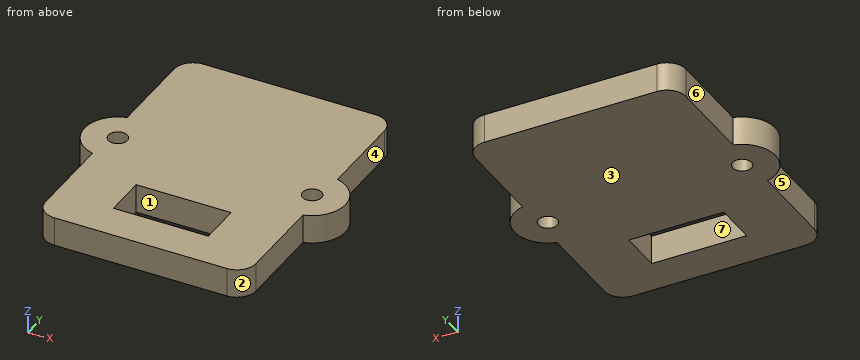
```python
from build123d import *

# Parameters (mm, degrees)
SKETCH2_R           = 1
SKETCH2_W           = 10
SKETCH2_H           = 4.5
BOSS_EXTRUDE2_DEPTH = 3.05


with BuildPart() as part:
    # Sketch2 → Boss-Extrude2 (new body)
    with BuildSketch(Plane.XY):
        with BuildLine():
            Line((-11.075, 15.855524923), (-11.075, 25.133587826))
            ThreePointArc((-11.075, 25.133587826), (-10.489213562, 26.547801388), (-9.075, 27.133587826))
            Line((-9.075, 27.133587826), (9.075, 27.133587826))
            ThreePointArc((9.075, 27.133587826), (10.489213562, 26.547801388), (11.075, 25.133587826))
            Line((11.075, 25.133587826), (11.075, 15.855524923))
            ThreePointArc((11.075, 15.855524923), (13.735, 12.45), (11.075, 9.044475077))
            Line((11.075, 9.044475077), (11.075, -0.233587826))
            ThreePointArc((11.075, -0.233587826), (10.489213562, -1.647801388), (9.075, -2.233587826))
            Line((9.075, -2.233587826), (-9.075, -2.233587826))
            ThreePointArc((-9.075, -2.233587826), (-10.489213562, -1.647801388), (-11.075, -0.233587826))
            Line((-11.075, -0.233587826), (-11.075, 9.044475077))
            ThreePointArc((-11.075, 9.044475077), (-13.735, 12.45), (-11.075, 15.855524923))
        make_face()
        with Locations((-10.225, 12.45)):
            Circle(SKETCH2_R, mode=Mode.SUBTRACT)
        with Locations(Location((10.225, 12.45, 0), (0, 0, 180))):
            Circle(SKETCH2_R, mode=Mode.SUBTRACT)
        with Locations((0, 4.016412174)):
            Rectangle(SKETCH2_W, SKETCH2_H, mode=Mode.SUBTRACT)
    extrude(amount=BOSS_EXTRUDE2_DEPTH)


solid = part.part
```
Geometry: final body of the model. Coordinates: model frame, mm. Face numbers are marked on the shaded views. A direction names the side the tool comes from. Give positions to 0.01 mm unless a question says otherwise; leave off trailing zeros. Loops run counter-clockwise (first coordinate to the right, second up) from the corner with the lowest first, then second, coordinate; pieces in that order, holes last. Notation, with made-up numbers: (39, 22.25) -> (62, 22.25) arc R21 cw to (62, 32.25) -> close; hole circle Ø3 at (80, 21). An arc over 180 degrees is marked (long way). Use one line per item in the form item = value.
Item 1: Pin query (flat end, axial travel): P1, Ø1.5, axis at y = 4.5, z = 1, coming from the -X side (3 decimals); P2, Ø2, axis at x = 3.5, y = 2.5, coming from the +Z side; P3, Ø1.5, axis at y = 5, z = 2, coming from the +X side (3 decimals). Return the tip coordinate at first contact, or that it passes through.
A:
P1 = -11.075
P2 = 3.05
P3 = 11.075
Item 2: Line query: probe 1 along Y at (x, z) = (4.25, 0.95); probe 2 along X at (y, z) = (7.5, 2.7) (3 decimals). Output: solid intervals per line, ascending.
A:
probe_1 = -2.23 to 1.77, 6.27 to 27.13
probe_2 = -11.075 to 11.075
Item 3: Draft query along X for the marked faces 1, 2 and 3. Return one class per face: pulls with the +X half, pulls with the -X half, needs draft (parallel to the pull), parting line crosses it, or undercut.
A:
face_1 = undercut
face_2 = pulls with the +X half
face_3 = needs draft
Item 4: Section query C-C on z = 1.25. Output: boundary loops of the cut face in (x, y) (3 decimals), and give its area (3 significant figures).
A:
outline = (-11.075, -0.234) arc R2 ccw to (-9.075, -2.234) -> (9.075, -2.234) arc R2 ccw to (11.075, -0.234) -> (11.075, 9.044) arc R3.51 ccw to (11.075, 15.856) -> (11.075, 25.134) arc R2 ccw to (9.075, 27.134) -> (-9.075, 27.134) arc R2 ccw to (-11.075, 25.134) -> (-11.075, 15.856) arc R3.51 ccw to (-11.075, 9.044) -> close; hole circle Ø2 at (-10.225, 12.45); hole (-5, 1.766) -> (5, 1.766) -> (5, 6.266) -> (-5, 6.266) -> close; hole circle Ø2 at (10.225, 12.45)
area = 623 mm^2
Item 5: Access query for the marked faces 4, 5, 6 and 7. Directions: +Z, -Z, +X, -X, +Y, -Y. A direction counts if a zero-diameter tool reaches every point of the face in a straight line with its end or side. Return the directions, or none.
A:
face_4 = +Z, -Z, +X, +Y
face_5 = +Z, -Z, -X, -Y
face_6 = +Z, -Z, -X, +Y
face_7 = +Z, -Z
Item 6: Section query B-B on y = 12.45. Output: boundary loops of the cut face in (x, z) (3 decimals).
A:
outline = (-13.735, 0) -> (-11.225, 0) -> (-11.225, 3.05) -> (-13.735, 3.05) -> close; (-9.225, 0) -> (9.225, 0) -> (9.225, 3.05) -> (-9.225, 3.05) -> close; (11.225, 0) -> (13.735, 0) -> (13.735, 3.05) -> (11.225, 3.05) -> close
Item 7: Section query A-A on x = 4.25. Output: boundary loops of the cut face in (y, z), and give its area (3 significant figures).
A:
outline = (-2.23, 0) -> (1.77, 0) -> (1.77, 3.05) -> (-2.23, 3.05) -> close; (6.27, 0) -> (27.13, 0) -> (27.13, 3.05) -> (6.27, 3.05) -> close
area = 75.8 mm^2
Item 8: Section query D-D on y = 17.75. Output: boundary loops of the cut face in (x, z) (3 decimals), and give its area (3 significant figures).
A:
outline = (-11.075, 0) -> (11.075, 0) -> (11.075, 3.05) -> (-11.075, 3.05) -> close
area = 67.6 mm^2
